Solid Edge part; units mm, degrees
sketch "Sketch1" plane through (0, 0, 0) normal (0, 0, 1) x (1, 0, 0)
  circle A0 centre (0, 0) radius 4.5964
extrude "Protrusion1" add sketch "Sketch1" along normal blind 3.048
sketch "Sketch2" plane through (0, 0, 0) normal (0, 0, -1) x (1, 0, 0)
  circle A0 centre (0, 0) radius 2.413
extrude "Protrusion2" add sketch "Sketch2" along normal blind 38.1
sketch "Sketch3" plane through (0, 0, -38.1) normal (0, 0, -1) x (1, 0, 0)
  circle A0 centre (0, 0) radius 2.4127
extrude "Cutout1" cut sketch "Sketch3" against normal blind 9.525 flip side to cut
chamfer "Chamfer_1" distance 0.3619 angle 45 1 edges at (-2.4127, 0, -38.1)
sketch "Sketch4" plane through (0, 0, 3.048) normal (0, 0, 1) x (1, 0, 0)
  line L0 (-2.3294, 3.9624) -> (2.3294, 3.9624)
extrude "Cutout2" cut sketch "Sketch4" against normal up to next material side at (0, 4.0124, 3.048)
pattern_circular "Pattern1" count 6 over 360 about axis through (0, 0, 3.048) along (0, 0, 1) of "Cutout2"
properties part number "185522"
Here's how the part is built. I have some questions about the finished solid (model axes, mm). A direction names the side the tool comes from. Give positions to 0.01 mm unless a question says otherwise; leave off trailing zeros. Order: outer loops, then holes, each group sorted by start corner. A loop starts at its lowest first (then second) coordinate and runs counter-clockwise, first axis right, second up. Notation, with made-up numbers: (81, 82.25) -> (117, 82.25) arc R20 ccw to (117, 89.25) -> close; hole circle Ø4 at (70, -34). An arc over 180 degrees is marked (long way). One line per item, written item: value. Start each with the question number.
1. I need wall thicknesses on probe 1 along Z at (x, y) = (1.5, 3); probe 2 along Y at (x, z) = (-0.75, -9); probe 3 along X at (y, z) = (-0.5, -18). Which ranges of each line are inside material? Lowest first, please. Write a range as from..to.
2. Imagine slicing it at B-B, the plane z = -2. List the corners of the cut face in (x, y) for me, plus the area to 3 significant figures.
3. Imagine slicing it at C-C, the plane y = 3. List the corners of the cut face in (x, z) for me, plus the area to 3 significant figures.
4. For faces 1 (the face through (2, 2, 0)), 2 (the face through (0, 0, 3.048)), which set-ups out of +Z, -Z, +X, -X, +Y, -Y let a thin tool reach every point of the face, with its end or its side?
5. Will these pins go through, and if not, where does the flat tip stop? pin 1 Ø3 at (y, z) = (3, -3.5) entering from +X; pin 2 Ø2 at (y, z) = (0.5, -29.5) entering from -X; pin 3 Ø3 at (y, z) = (3, -16.5) entering from -X.
Values follow:
1. probe 1: z = 0..3.05
1. probe 2: y = -2.29..2.29
1. probe 3: x = -2.36..2.36
2. outline: circle Ø4.83 at (0, 0)
2. area: 18.3 mm2
3. outline: (-2.84, 0) -> (2.84, 0) -> (2.84, 3.05) -> (-2.84, 3.05) -> close
3. area: 17.3 mm2
4. face 1: -Z
4. face 2: +Z, +X, -X, +Y, -Y
5. pin 1: stops at x = 1.89
5. pin 2: stops at x = -2.41
5. pin 3: stops at x = -1.89
